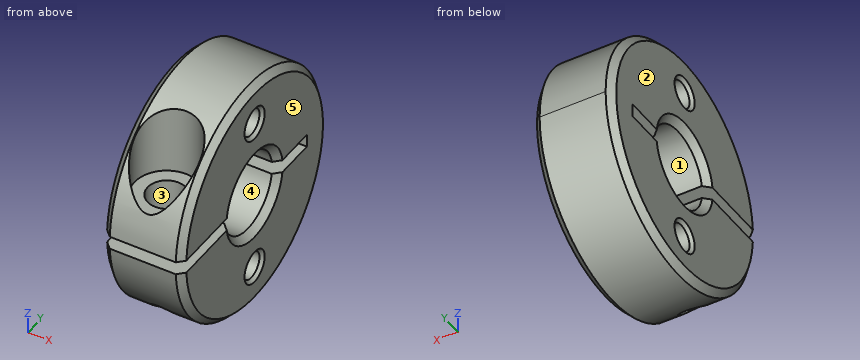
Autodesk Inventor part; units mm, degrees
ref_plane "body_screw_XY" through (0, -6, 3) normal (0, 0, 1) x (1, 0, 0)
ref_plane "body_screw_YZ" through (0, -6, 3) normal (1, 0, 0) x (0, 1, 0)
ref_plane "body_screw_ZX" through (0, -6, 3) normal (0, 1, 0) x (0, 0, 1)
sketch "Sketch_1" plane through (0, 0, 0) normal (0, 0, 1) x (1, 0, 0)
  line L0 (3, 0) -> (-3, 0)
  line L1 (-3, 8.5) -> (-3, 3.5)
  line L2 (-3, 3.5) -> (-2.5, 3)
  line L3 (-2.5, 3) -> (2.5, 3)
  line L4 (2.5, 3) -> (3, 3.5)
  line L5 (3, 3.5) -> (3, 8.5)
  line L6 (3, 8.5) -> (2.5, 9)
  line L7 (2.5, 9) -> (-2.5, 9)
  line L8 (-2.5, 9) -> (-3, 8.5)
revolve "Revolution1" add sketch "Sketch_1" angle 360 about axis through (3, 0, 0) along (1, 0, 0)
sketch "Sketch_2" plane through (0, 0, 0) normal (1, 0, 0) x (0, 1, 0)
  line L0 (-9, 0.5) -> (-9, -0.5)
  line L1 (-9, -0.5) -> (6.5, -0.5)
  line L2 (6.5, -0.5) -> (6.5, 0.5)
  line L3 (6.5, 0.5) -> (-9, 0.5)
extrude "Extrusion1" cut sketch "Sketch_2" along normal mid plane 6
sketch "Sketch_3" plane through (0, 0, 0) normal (1, 0, 0) x (0, 1, 0)
  line L0 (-6, 9) -> (-6, 0)
  line L1 (-6, 0) -> (-7.45, 0)
  line L2 (-7.45, 0) -> (-7.45, 3)
  line L3 (-7.45, 3) -> (-8.45, 3)
  line L4 (-8.45, 3) -> (-8.45, 9)
  line L5 (-8.45, 9) -> (-6, 9)
  line L6 (-6, 9) -> (-6, 0)
revolve "Revolution2" cut sketch "Sketch_3" angle 360 about axis through (0, -6, 9) along (0, 0, 1)
sketch "Sketch_4" plane through (0, 0, 0) normal (1, 0, 0) x (0, 1, 0)
  line L0 (-6, -9.5) -> (-6, -0.5)
  line L1 (-6, -0.5) -> (-4.75, -0.5)
  line L2 (-4.75, -0.5) -> (-4.9935, -0.7435)
  line L3 (-4.9935, -0.7435) -> (-4.9935, -9.5)
  line L4 (-4.9935, -9.5) -> (-6, -9.5)
  line L5 (-6, -9.5) -> (-6, -0.5)
revolve "Revolution3" cut sketch "Sketch_4" angle 360 about axis through (0, -6, -9.5) along (0, 0, -1)
thread "Thread1"
sketch "Sketch_7" plane through (0, 0, -6) normal (0, 0, 1) x (1, 0, 0)
  line L0 (3, 0) -> (-3, 0)
  line L1 (-3, 0) -> (-3, 1.25)
  line L2 (-3, 1.25) -> (-2.7565, 1.0065)
  line L3 (-2.7565, 1.0065) -> (2.7565, 1.0065)
  line L4 (2.7565, 1.0065) -> (3, 1.25)
  line L5 (3, 1.25) -> (3, 0)
  line L6 (3, 0) -> (-3, 0)
revolve "Revolution4" cut sketch "Sketch_7" angle 360 about axis through (3, 0, -6) along (1, 0, 0)
thread "Thread2"
sketch "Sketch_8" plane through (0, 0, 6) normal (0, 0, 1) x (1, 0, 0)
  line L0 (3, 0) -> (-3, 0)
  line L1 (-3, 0) -> (-3, 1.25)
  line L2 (-3, 1.25) -> (-2.7565, 1.0065)
  line L3 (-2.7565, 1.0065) -> (2.7565, 1.0065)
  line L4 (2.7565, 1.0065) -> (3, 1.25)
  line L5 (3, 1.25) -> (3, 0)
  line L6 (3, 0) -> (-3, 0)
revolve "Revolution5" cut sketch "Sketch_8" angle 360 about axis through (3, 0, 6) along (1, 0, 0)
thread "Thread3"
ref_plane "body_screw_XY" through (0, -6, 3) normal (0, 0, 1) x (1, 0, 0)
ref_plane "body_screw_YZ" through (0, -6, 3) normal (1, 0, 0) x (0, 1, 0)
ref_plane "body_screw_ZX" through (0, -6, 3) normal (0, 1, 0) x (0, 0, 1)
properties part number "SCSWJ6-6_b"
Input: part model. Units: mm. Frame: model coordinates. Face numbers are marked on the shaded views. A direction names the side the tool comes from. Round coordinates to 2 decimals unless told otherwise and drop trailing zeros. Order: outer loops, then holes, each group sorted by start corner. A loop starts at its lowest first (then second) coordinate and runs counter-clockwise, first axis right, second up. Notation, with made-up numbers: (80.5, 76) - (84.5, 76) arc R18 cw to (84.5, 88) - close; hole circle Ø3 at (59, 21). An arc over 180 degrees is marked (long way). Answer as a JSON object with one key per item and string values. Group by question number.
(1) Draft query along Y for the marked faces 4 and 5. Return one class per face: released by +Y, released by -Y, zero draft, split by the parting line, or undercut.
(2) Cut plane B-B (x = 1.75). Return loops of the section in (y, z).
(3) Pin query (flat end, axial travel): P1, Ø1.1, axis at x = -1, y = 4, coming from the +Z side; P2, Ø3, axis at x = 0, y = -6, coming from the -Z side; P3, Ø3, axis at x = 1, z = -6.5, coming from the -Y side. Return the tip coordinate at first contact, or that it passes through.
(4) Cut plane A-A (y = 0). Count the separate pieces of the cut face and the enclosed holes in it, then the cut area to 3 significant figures.
(5) Reachability of the marked faces 1, 2 and 3 from +Z, -Z, +X, -X, +Y, -Y: full face, straight path, thin tool, end or side. Return the list, or none.
(6) Material intervals for probe 1 along Z at (x, y) = (0.4, 0); probe 2 along Y at (x, z) = (-0.5, -5.25); probe 3 along Z at (x, y) = (0.25, -0.75), sorted ascending. Write a range as from..to.
Here are the results:
{
 "1": {"face 4": "undercut", "face 5": "zero draft"},
 "2": {"outline": "(-8.99, -0.5) arc R9 ccw (long way) to (-4.29, 7.91) - (-4.29, 3) - (-7.71, 3) - (-7.71, 4.64) arc R9 ccw to (-8.99, 0.5) - (-2.96, 0.5) arc R3 cw to (2.96, 0.5) - (6.5, 0.5) - (6.5, -0.5) - (2.96, -0.5) arc R3 cw to (-2.96, -0.5) - close; hole circle Ø2.01 at (0, -6); hole circle Ø2.01 at (0, 6)"},
 "3": {"P1": "stops at z = 8.31", "P2": "stops at z = -7.79", "P3": "stops at y = -7.48"},
 "4": {"separate pieces": "4", "enclosed holes": "0", "area": "46.6 mm^2"},
 "5": {"face 1": "+X, -X", "face 2": "+Z, -Z, -X, +Y, -Y", "face 3": "+Z"},
 "6": {"probe 1": "z = -9..-7.01, -4.99..-3, 3..4.99, 7.01..9", "probe 2": "y = -7.31..-6.87, -5.13..-0.67, 0.67..7.31", "probe 3": "z = -8.97..-6.67, -5.33..-2.9, 2.9..5.33, 6.67..8.97"}
}
